For this review, use the dimensioned drawing (mm, ordinates from the lowest corner) and the shaded views. A direction names the side the tool comes from. Give positions to 0.01 mm unless a question says otherwise; leave off trailing zeros. Write each loop counter-clockwise with the first axis right and the second up, starting at its lowest first coordinate (ties: lowest second). Pieces come first, ordered by that corner, then holes.
1) Wall thickness on line 1 along Z through (x, y) = (125, 76.5); line 2 along Y through (x, z) = (38, 45); line 3 along Z through (x, y) = (116.5, 68.5): over which ranges is each line inside the solid? List them lowest first.
2) We need section C-C on y = 17. Give the boundary of the cut face in (x, z), and give its area (3 significant figures).
3) We need section B-B on z = 16. Give the boundary of the cut face in (x, y).
4) We need section D-D on z = 55. Give the boundary of the cut face in (x, y).
5) Machinability: for the marked faces 1, 2 and 3, which of the approach directions +Z, -Z, +X, -X, +Y, -Y give a long, thin tool a straight path to every point of the face, cutting with its end or side? Answer none if there is none.
6) For P1, Ø15, axis at x = 22, z = 53, coming from the -Y side; P2, Ø15, axis at x = 16, y = 45.5, coming from the +Z side; P3, Ø15.5, axis at y = 52, z = 59, coming from the -X side, all flat-tipped, find the tip position at first contact; note any pin that passes through.
7) We need section A-A on x = 125. Give the boundary of the cut face in (y, z).
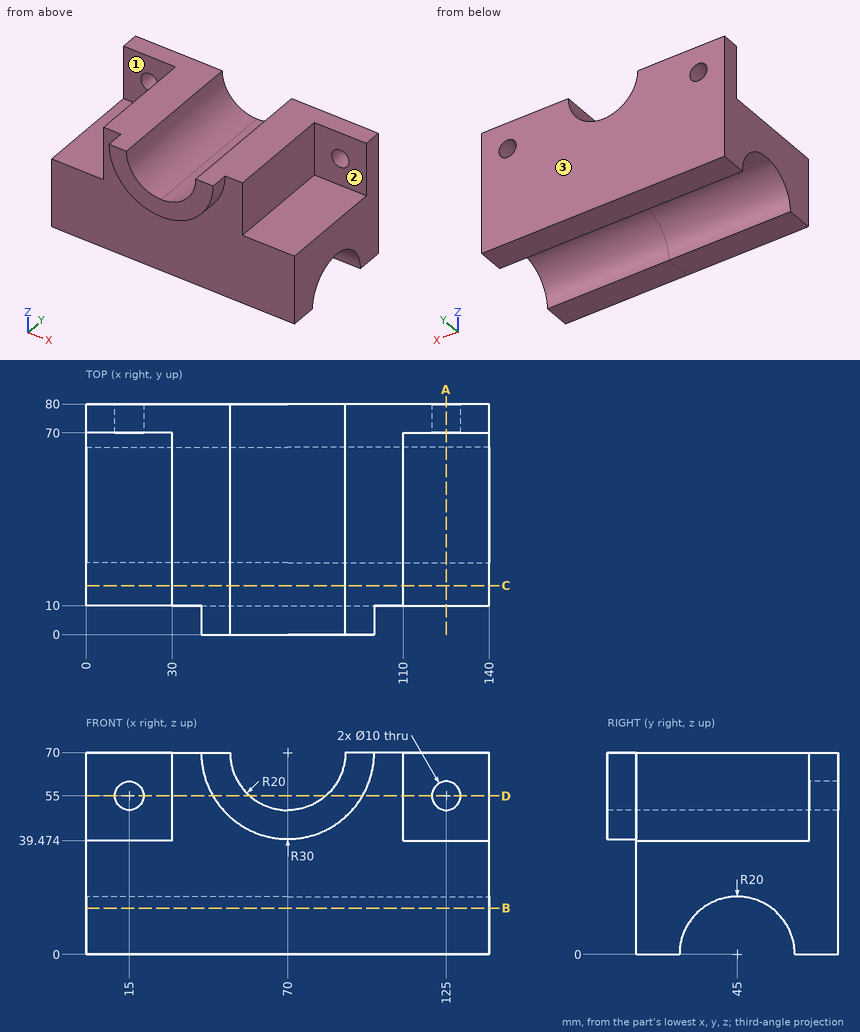
Results list:
1. line 1: z = 0 to 50, 60 to 70
1. line 2: y = 10 to 80
1. line 3: z = 0 to 39.47
2. outline: (0, 0) - (140, 0) - (140, 39.47) - (110, 39.47) - (110, 70) - (90, 70) arc R20 cw to (50, 70) - (30, 70) - (30, 39.47) - (0, 39.47) - close
2. area: 7,340 mm2
3. outline: (0, 10) - (140, 10) - (140, 33) - (0, 33) - close; (0, 57) - (140, 57) - (140, 80) - (0, 80) - close
4. outline: (0, 70) - (10, 70) - (10, 80) - (0, 80) - close; (20, 70) - (30, 70) - (30, 10) - (44.02, 10) - (44.02, 0) - (56.77, 0) - (56.77, 80) - (20, 80) - close; (83.23, 0) - (95.98, 0) - (95.98, 10) - (110, 10) - (110, 70) - (120, 70) - (120, 80) - (83.23, 80) - close; (130, 70) - (140, 70) - (140, 80) - (130, 80) - close
5. face 1: +Z, -X, -Y
5. face 2: +Z, +X, -Y
5. face 3: +Z, -Z, +X, -X, +Y
6. P1: stops at y = 70
6. P2: stops at z = 39.47
6. P3: stops at x = 30
7. outline: (10, 0) - (25, 0) arc R20 cw to (65, 0) - (80, 0) - (80, 50) - (70, 50) - (70, 39.47) - (10, 39.47) - close; (70, 60) - (80, 60) - (80, 70) - (70, 70) - close
